Could you check a few things on this model? Use its own coordinates, in mm. A direction names the side the tool comes from. Coordinates: 2 decimals unless noted, no trailing zeros. Write each loop counter-clockwise with the first axis right and the second up, starting at its lowest first coordinate (ties: lowest second). Pieces come first, ordered by that corner, then holes.
Item 1: I want a section at B-B on z = 0. Please give me the cut outline in (x, y).
Item 2: For P1, Ø2.5, axis at y = 8.5, z = -0.5, coming from the +X side; P2, Ø2.5, axis at y = 12, z = -0.5, coming from the -X side; P3, Ø4, axis at y = 9.5, z = 0, coming from the +X side, each with a flat end and sliding along its axis, tell me the tip position at first contact or that it passes through.
Item 3: I want a section at D-D on y = 7. Please give me the cut outline in (x, z), then the cut area to 3 significant figures.
Item 4: If I drill on probe 1 along Z at (x, y) = (2, 13.75); probe 2 along Z at (x, y) = (-3, 10.25); probe 3 along X at (y, z) = (8, 4.25), over which ranges is the centre line in solid material (lowest first)?
Item 5: I want a section at A-A on y = 12. Please give me the cut outline in (x, z).
Item 6: Thinking about a two-plate mould opening in Z: for faces 4 (the flat face through (0, 7, 6)), 5 (the flat face through (-16.2, 4, -3)), 6 (the flat face through (-7.7, 10, -2)), which applies, +Z half, -Z half, draft (parallel to the pull), parting line (faces both ways), or undercut?
Item 7: Which directions (+Z, -Z, +X, -X, +Y, -Y) give clear straight access to the entire face, cutting with the end or side of a thin tool? Please do faces 1 (the flat face through (8, 12, -3.354)), 2 (the cylindrical face through (-12, 3, 0)), 3 (the flat face through (0.2, 10, 2)).
Item 8: I want a section at C-C on z = -3. Please give me the cut outline in (x, y).
from build123d import *

# Parameters (mm, degrees)
SKETCH_1_W          = 32.4
SKETCH_1_H          = 12
EXTRUDE_1_DEPTH     = 10
SKETCH_4_R          = 4
CUT_EXTRUDE_2_DEPTH = 8.5
SKETCH_7_R          = 3.4
CUT_EXTRUDE_3_DEPTH = 7.9
SKETCH_8_R          = 4.5
CUT_EXTRUDE_4_DEPTH = 16
SKETCH_9_W          = 32.4
SKETCH_9_H          = 2.645898034
EXTRUDE_2_DEPTH     = 5
EXTRUDE_3_DEPTH     = 5
EXTRUDE_4_DEPTH     = 5


with BuildPart() as part:
    # 草圖1 → 填料-伸長1 (new body)
    with BuildSketch(Plane(origin=(0, 0, 0), x_dir=(1, 0, 0), z_dir=(0, 1, 0))):
        Rectangle(SKETCH_1_W, SKETCH_1_H)
    extrude(amount=EXTRUDE_1_DEPTH)

    # 草圖4 → 除料-伸長2 (cut)
    with BuildSketch(Plane.ZY.offset(16.2)):
        with Locations((0, 7)):
            Circle(SKETCH_4_R)
    extrude(amount=-CUT_EXTRUDE_2_DEPTH, mode=Mode.SUBTRACT)

    # 草圖7 → 除料-伸長3 (cut)
    with BuildSketch(Plane.ZY.offset(7.7)):
        with Locations((0, 7)):
            Circle(SKETCH_7_R)
    extrude(amount=-CUT_EXTRUDE_3_DEPTH, mode=Mode.SUBTRACT)

    # 草圖8 → 除料-伸長4 (cut)
    with BuildSketch(Plane(origin=(16.2, 0, 0), x_dir=(0, 0, -1), z_dir=(1, 0, 0))):
        with Locations((0, 7)):
            Circle(SKETCH_8_R)
    extrude(amount=-CUT_EXTRUDE_4_DEPTH, mode=Mode.SUBTRACT)

    # 草圖9 → 填料-伸長2 (add)
    with BuildSketch(Plane(origin=(0, 10, 0), x_dir=(1, 0, 0), z_dir=(0, 1, 0))):
        with Locations((0, 4.677050983)):
            Rectangle(SKETCH_9_W, SKETCH_9_H)
    extrude(amount=EXTRUDE_2_DEPTH)

    # 草圖10 → 填料-伸長3 (add)
    with BuildSketch(Plane(origin=(0, 10, 0), x_dir=(1, 0, 0), z_dir=(0, 1, 0))):
        Polygon((-16.2, 3.372532617), (-16.2, 2.685476071), (-7.7, 2.645751311), (-7.7, 1.6), (0.2, 1.6), (0.2, 3.354101966), align=None)
    extrude(amount=EXTRUDE_3_DEPTH)

    # 草圖11 → 填料-伸長4 (add)
    with BuildSketch(Plane(origin=(0, 10, 0), x_dir=(1, 0, 0), z_dir=(0, 1, 0))):
        Polygon((-16.2, -2.660675208), (-16.2, -6), (16.2, -6), (16.2, -3.354101966), (0.2, -3.354101966), (0.2, -1.6), (-7.7, -1.6), (-7.7, -2.645751311), align=None)
    extrude(amount=EXTRUDE_4_DEPTH)


solid = part.part
Response values:
1. outline: (-16.2, 0) - (16.2, 0) - (16.2, 2.5) - (0.2, 2.5) - (0.2, 3.6) - (-7.7, 3.6) - (-7.7, 3) - (-16.2, 3) - close
2. P1: passes through
2. P2: stops at x = -7.7
2. P3: stops at x = 0.2
3. outline: (-16.2, -6) - (16.2, -6) - (16.2, -4.5) - (0.2, -4.5) - (0.2, -3.4) - (-7.7, -3.4) - (-7.7, -4) - (-16.2, -4) - close; (-16.2, 4) - (-7.7, 4) - (-7.7, 3.4) - (0.2, 3.4) - (0.2, 4.5) - (16.2, 4.5) - (16.2, 6) - (-16.2, 6) - close
3. area: 123 mm2
4. probe 1: z = -6 to -3.35, 3.35 to 6
4. probe 2: z = -6 to -1.6, 1.6 to 6
4. probe 3: x = -16.2 to 0.2
5. outline: (-16.2, -6) - (16.2, -6) - (16.2, -3.35) - (0.2, -3.35) - (0.2, -1.6) - (-7.7, -1.6) - (-7.7, -2.65) - (-16.2, -2.69) - close; (-16.2, 2.66) - (-7.7, 2.65) - (-7.7, 1.6) - (0.2, 1.6) - (0.2, 3.35) - (16.2, 3.35) - (16.2, 6) - (-16.2, 6) - close
6. face 4: +Z half
6. face 5: draft
6. face 6: undercut
7. face 1: +X, +Y
7. face 2: -X
7. face 3: +X
8. outline: (-16.2, 0) - (16.2, 0) - (16.2, 3.65) - (0.2, 3.65) - (0.2, 5.4) - (-7.7, 5.4) - (-7.7, 4.35) - (-16.2, 4.35) - close; (-16.2, 9.65) - (-7.7, 9.65) - (-7.7, 8.6) - (0.2, 8.6) - (0.2, 15) - (-16.2, 15) - close
